Work out the finished part from the listing and answer in its coordinate system (mm). A direction names the side the tool comes from. Give positions to 0.01 mm unless a question says otherwise; leave off trailing zeros. Order: outer loops, then holes, each group sorted by start corner. A loop starts at its lowest first (then second) coordinate and runs counter-clockwise, first axis right, second up.
```python
from build123d import *

# Parameters (mm, degrees)
SKETCH1_W           = 325
SKETCH1_H           = 75
BOSS_EXTRUDE1_DEPTH = 42.5
SKETCH2_R           = 1.5
CUT_EXTRUDE1_DEPTH  = 10
SKETCH3_W           = 10
SKETCH3_H           = 105
BOSS_EXTRUDE2_DEPTH = 120
SHELL1_START        = -32.5
SHELL1_OUTLINE_W    = 315
SHELL1_OUTLINE_H    = 80
SHELL1_OUTLINE_R    = 6.5
SHELL1_DEPTH        = 65
SHELL1_2_OUTLINE_R  = 6.5
SHELL1_2_DEPTH      = 55
SKETCH4_W           = 30
SKETCH4_H           = 15
CUT_EXTRUDE2_DEPTH  = 368.134171659
SKETCH5_R           = 2
CUT_EXTRUDE3_DEPTH  = 368.134171659


# Read off the part's stored shape, not the designer's step: Shell1
with BuildPart() as part:
    # Sketch1 → Boss-Extrude1 (new, symmetric)
    with BuildSketch(Plane(origin=(0, 0, 0), x_dir=(1, 0, 0), z_dir=(0, 1, 0))):
        Rectangle(SKETCH1_W, SKETCH1_H)
    extrude(amount=BOSS_EXTRUDE1_DEPTH, both=True)

    # Sketch2 → Cut-Extrude1 (cut)
    with BuildSketch(Plane.XY.offset(37.5)):
        with Locations((-50, 0)):
            Circle(SKETCH2_R)
        with Locations(Location((50, 0, 0), (0, 0, 180))):
            Circle(SKETCH2_R)
    extrude(amount=-CUT_EXTRUDE1_DEPTH, mode=Mode.SUBTRACT)

    # Sketch3 → Boss-Extrude2 (add)
    with BuildSketch(Plane(origin=(0, 42.5, 0), x_dir=(1, 0, 0), z_dir=(0, 1, 0))):
        with Locations((-157.5, 0)):
            Rectangle(SKETCH3_W, SKETCH3_H)
    boss_extrude2 = extrude(amount=BOSS_EXTRUDE2_DEPTH)

    # Mirror1: Boss-Extrude2 across plane
    add(boss_extrude2.mirror(Plane(origin=(0, 0, 0), x_dir=(0, 0, 1), z_dir=(1, 0, 0))))

    # Shell1 outline → Shell1 (cut)
    with BuildSketch(Plane.XY.offset(SHELL1_START)):
        with Locations((0, 2.5)):
            Rectangle(SHELL1_OUTLINE_W, SHELL1_OUTLINE_H)
        with Locations((-50, 0)):
            Circle(SHELL1_OUTLINE_R, mode=Mode.SUBTRACT)
        with Locations((50, 0)):
            Circle(SHELL1_OUTLINE_R, mode=Mode.SUBTRACT)
    extrude(amount=SHELL1_DEPTH, mode=Mode.SUBTRACT)

    # Shell1 2 outline → Shell1 2 (cut)
    with BuildSketch(Plane.XY.offset(SHELL1_START)):
        with Locations((50, 0)):
            Circle(SHELL1_2_OUTLINE_R)
        with Locations((-50, 0)):
            Circle(SHELL1_2_OUTLINE_R)
    extrude(amount=SHELL1_2_DEPTH, mode=Mode.SUBTRACT)

    # Sketch4 → Cut-Extrude2 (cut, through all)
    with BuildSketch(Plane(origin=(162.5, 0, 0), x_dir=(0, 0, -1), z_dir=(1, 0, 0))):
        Rectangle(SKETCH4_W, SKETCH4_H)
    extrude(amount=-CUT_EXTRUDE2_DEPTH, mode=Mode.SUBTRACT)

    # Sketch5 → Cut-Extrude3 (cut, through all)
    with BuildSketch(Plane(origin=(162.5, 0, 0), x_dir=(0, 0, -1), z_dir=(1, 0, 0))):
        with Locations((-47.5, 47.5)):
            Circle(SKETCH5_R)
        with Locations((47.5, 47.5)):
            Circle(SKETCH5_R)
        with Locations((47.5, 157.5)):
            Circle(SKETCH5_R)
        with Locations((-47.5, 157.5)):
            Circle(SKETCH5_R)
    extrude(amount=-CUT_EXTRUDE3_DEPTH, mode=Mode.SUBTRACT)


solid = part.part
```
1. The part is cut by section C-C (y = -15). Write down the section's boundary in (x, z), then the cut area to 3 significant figures.
Findings below:
outline: (-162.5, -37.5) - (162.5, -37.5) - (162.5, 37.5) - (-162.5, 37.5) - close; hole (-157.5, -32.5) - (157.5, -32.5) - (157.5, 32.5) - (-157.5, 32.5) - close
area: 3,900 mm2
2. Which of the six approach directions +Z, -Z, +X, -X, +Y, -Y give full straight-line access (tool end or side, diameter ignored) to faces 4 (the face through (158, 42.5, 45)), 5 (the face through (-56.494, 0.286, 27.43)), 6 (the face through (162.5, 59, 1)), 7 (the face through (-50, 0, 22.5)), 8 (the face through (158, 42.5, -45))?
Findings below:
face 4: +Z, +X, -X, -Y
face 5: none
face 6: +Z, -Z, +X, +Y, -Y
face 7: +Y
face 8: -Z, +X, -X, -Y
3. The mould has two halves that part along Y. Classify faces 1 (the face through (-2, -42.5, -1)), 2 (the face through (-152.5, 102, 1)), 3 (the face through (-157.5, 11, 0)): pulls with the +Y half, pulls with the -Y half, needs draft (parallel to the pull), parting line crosses it, or undercut.
Findings below:
face 1: pulls with the -Y half
face 2: needs draft
face 3: undercut
4. Given P1, Ø2, axis at x = -109, z = -11.5, coming from the +Y side; P2, Ø10, axis at x = 61, y = 23, coming from the -Z side; P3, Ø2.5, axis at x = -49.5, y = 0, coming from the +Z side, each flat-ended and moving along its own axis, determine where each tip first touches the part or whether it passes through.
Findings below:
P1: stops at y = -37.5
P2: stops at z = -37.5
P3: stops at z = 37.5
5. The part is cut by section A-A (z = -4). Write down the section's boundary in (x, y), then the cut area to 4 significant figures.
Findings below:
outline: (-162.5, -42.5) - (162.5, -42.5) - (162.5, -7.5) - (157.5, -7.5) - (157.5, -37.5) - (-157.5, -37.5) - (-157.5, -7.5) - (-162.5, -7.5) - close; (-162.5, 7.5) - (-157.5, 7.5) - (-157.5, 42.5) - (-152.5, 42.5) - (-152.5, 162.5) - (-162.5, 162.5) - close; (152.5, 42.5) - (157.5, 42.5) - (157.5, 7.5) - (162.5, 7.5) - (162.5, 162.5) - (152.5, 162.5) - close
area: 4,675 mm2
6. The part is cut by section D-D (x = 81.5). Write down the section's boundary in (y, z), then the cut area to 4 significant figures.
Findings below:
outline: (-42.5, -37.5) - (42.5, -37.5) - (42.5, -32.5) - (-37.5, -32.5) - (-37.5, 32.5) - (42.5, 32.5) - (42.5, 37.5) - (-42.5, 37.5) - close
area: 1,175 mm2
7. The part is cut by section B-B (y = 79). Write down the section's boundary in (x, z), then the cut area to 3 significant figures.
Findings below:
outline: (-162.5, -52.5) - (-152.5, -52.5) - (-152.5, 52.5) - (-162.5, 52.5) - close; (152.5, -52.5) - (162.5, -52.5) - (162.5, 52.5) - (152.5, 52.5) - close
area: 2,100 mm2
8. Straight lines are drawn through the part: probe 1 along Y at (x, z) = (50, 30); probe 2 along Y at (x, z) = (157, -47); probe 3 along Z at (x, y) = (155, 157.5). For each, find the intervals that lie inside material, in ascending order.
Findings below:
probe 1: y = -42.5 to -37.5, -6.5 to -1.5, 1.5 to 6.5
probe 2: y = 42.5 to 45.56, 49.44 to 155.56, 159.44 to 162.5
probe 3: z = -52.5 to -49.5, -45.5 to 45.5, 49.5 to 52.5
